from build123d import *

# Parameters (mm, degrees)
SKETCH1_R             = 6.477
BOSS_EXTRUDE1_DEPTH   = 5.08
BOSS_EXTRUDE1_2_DEPTH = 5.08
SKETCH2_R             = 6.35
BOSS_EXTRUDE2_DEPTH   = 12.7
SKETCH3_R             = 9.652
CUT_EXTRUDE1_DEPTH    = 3.81
SKETCH5_R             = 3.175


with BuildPart() as part:
    # Sketch1 → Boss-Extrude1 (new, symmetric)
    with BuildSketch(Plane(origin=(0, 0, 0), x_dir=(1, 0, 0), z_dir=(0, 1, 0))):
        with BuildLine():
            Line((-46.355, -19.05), (-46.355, -9.651164438))
            ThreePointArc((-46.355, -9.651164438), (-38.1, 12.7), (-29.845, -9.651164438))
            Line((-29.845, -9.651164438), (-29.845, -19.05))
            ThreePointArc((-29.845, -19.05), (-38.1, -27.305), (-46.355, -19.05))
        make_face()
        with Locations(Location((-38.1, 0, 0), (0, 0, 270))):
            Circle(SKETCH1_R, mode=Mode.SUBTRACT)
    extrude(amount=BOSS_EXTRUDE1_DEPTH, both=True)



with BuildPart() as body_2:
    # Sketch1 → Boss-Extrude1 2 (new, symmetric)
    with BuildSketch(Plane(origin=(0, 0, 0), x_dir=(1, 0, 0), z_dir=(0, 1, 0))):
        with BuildLine():
            Line((29.845, -19.05), (29.845, -9.651164438))
            ThreePointArc((29.845, -9.651164438), (38.1, 12.7), (46.355, -9.651164438))
            Line((46.355, -9.651164438), (46.355, -19.05))
            ThreePointArc((46.355, -19.05), (38.1, -27.305), (29.845, -19.05))
        make_face()
        with Locations(Location((38.1, 0, 0), (0, 0, 90))):
            Circle(SKETCH1_R, mode=Mode.SUBTRACT)
    extrude(amount=BOSS_EXTRUDE1_2_DEPTH, both=True)


with BuildPart() as part_1:
    add(part.part)

    add(body_2.part)  # Boss-Extrude2 merges body 2
    # Sketch2 → Boss-Extrude2 (add)
    with BuildSketch(Plane.XZ.offset(5.08)):
        with Locations(Location((-38.1, 19.05, 0), (0, 0, 270))):
            Circle(SKETCH2_R)
        with Locations(Location((38.1, 19.05, 0), (0, 0, 270))):
            Circle(SKETCH2_R)
    extrude(amount=BOSS_EXTRUDE2_DEPTH)

    # Sketch3 → Cut-Extrude1 (cut)
    with BuildSketch(Plane(origin=(0, 5.08, 0), x_dir=(1, 0, 0), z_dir=(0, 1, 0))):
        with Locations(Location((-38.1, 0, 0), (0, 0, 270))):
            Circle(SKETCH3_R)
        with Locations(Location((38.1, 0, 0), (0, 0, 270))):
            Circle(SKETCH3_R)
    extrude(amount=-CUT_EXTRUDE1_DEPTH, mode=Mode.SUBTRACT)

    # Sweep1: sweep along a path in Sketch6
    with BuildLine(Plane(origin=(0, 0, 0), x_dir=(1, 0, 0), z_dir=(0, 1, 0))) as sweep1_path:
        Line((38.1, 12.192), (38.1, 44.45))
        ThreePointArc((38.1, 44.45), (35.310192091, 51.185192091), (28.575, 53.975))
        Line((28.575, 53.975), (-28.575, 53.975))
        ThreePointArc((-28.575, 53.975), (-35.310192091, 51.185192091), (-38.1, 44.45))
        Line((-38.1, 44.45), (-38.1, 12.192))
    # Sketch5 → Sweep1 (sweep)
    with BuildSketch(Plane.XY.offset(-12.192)):
        with Locations((38.1, 0)):
            Circle(SKETCH5_R)
    sweep(path=sweep1_path.line)


solid = part_1.part
The listing builds one solid part. Answer for the finished solid, in the listing's coordinates (mm). A direction names the side the tool comes from. Give positions to 0.01 mm unless a question says otherwise; leave off trailing zeros. Write each loop counter-clockwise with the first axis right and the second up, starting at its lowest first coordinate (ties: lowest second). Pieces come first, ordered by that corner, then holes.
1) Section D-D (x = 6) is taken. Write down the section's boundary in (y, z) (3 decimals), and give its area (3 significant figures).
2) Find the intervals of material crossed by L1, parallel to X at y = 2.8, z = 0; L2, parallel to Z at x = -38.1, y = -3.25 (3 decimals); L3, parallel to X at y = -2, z = 0, in increasing order.
3) Section A-A (z = 17) is taken. Write down the section's boundary in (x, y) (3 decimals).
4) A tool of negligible diameter and unlimited length cuts with its end or side. For faces 1 (the face through (31.8, 1.27, -2.3)), 2 (the face through (-0.4, -0.1, -50.8)), 3 (the face through (31.9, -11.34, 20.43)), 4 (the face through (29.845, 0, 14)), from which of +Z, -Z, +X, -X, +Y, -Y can it reach the whole face along a straight path? Write none if from no direction.
5) Given P1, Ø3, axis at y = 0.5, z = 13, coming from the +X side (3 decimals); P2, Ø10.5, axis at y = 1.5, z = 13.5, coming from the +X side; P3, Ø10, axis at x = -26.5, y = -8.5, coming from the -Z side, each flat-ended and moving along its own axis, determine where each tip first touches the part or whether it passes through.
6) Section B-B (y = 0) is taken. Write down the section's boundary in (x, z) (3 decimals).
7) For a pull along X with two mould halves and no side action, classify faces 5 (the face through (-38, 5.08, 11)), 6 (the face through (-47.522, 3.202, -2.092)), 7 (the face through (46.355, 0, 14)), 8 (the face through (-46.355, 0, 14)) as pulls with the +X half, pulls with the -X half, needs draft (parallel to the pull), parting line crosses it, or undercut.
8) Section C-C (z = 0) is taken. Write down the section's boundary in (x, y), and give its area (3 significant figures).
Response:
1. outline: circle Ø6.35 at (0, -53.975)
1. area: 31.7 mm2
2. L1: x = -50.8 to -47.75, -28.45 to -25.4, 25.4 to 28.45, 47.75 to 50.8
2. L2: z = -12.7 to -6.477, 6.477 to 27.305
2. L3: x = -50.8 to -44.58, -31.62 to -25.4, 25.4 to 31.62, 44.58 to 50.8
3. outline: (-46.355, -5.08) - (-44.11, -5.08) - (-44.11, -17.78) - (-32.09, -17.78) - (-32.09, -5.08) - (-29.845, -5.08) - (-29.845, 5.08) - (-46.355, 5.08) - close; (29.845, -5.08) - (32.09, -5.08) - (32.09, -17.78) - (44.11, -17.78) - (44.11, -5.08) - (46.355, -5.08) - (46.355, 5.08) - (29.845, 5.08) - close
4. face 1: +Y
4. face 2: none
4. face 3: -Y
4. face 4: +Z, +Y, -Y
5. P1: stops at x = 46.355
5. P2: stops at x = 47.76
5. P3: stops at z = -9.9
6. outline: (-46.355, 9.651) arc R12.7 ccw to (-41.275, -12.297) - (-41.275, -44.45) arc R12.7 ccw to (-28.575, -57.15) - (28.575, -57.15) arc R12.7 ccw to (41.275, -44.45) - (41.275, -12.297) arc R12.7 ccw to (46.355, 9.651) - (46.355, 19.05) arc R8.255 ccw to (29.845, 19.05) - (29.845, 9.651) arc R12.7 ccw to (34.925, -12.297) - (34.925, -44.45) arc R6.35 cw to (28.575, -50.8) - (-28.575, -50.8) arc R6.35 cw to (-34.925, -44.45) - (-34.925, -12.297) arc R12.7 ccw to (-29.845, 9.651) - (-29.845, 19.05) arc R8.255 ccw to (-46.355, 19.05) - close; hole circle Ø12.954 at (-38.1, 0); hole circle Ø12.954 at (38.1, 0)
7. face 5: needs draft
7. face 6: undercut
7. face 7: pulls with the +X half
7. face 8: pulls with the -X half
8. outline: (-50.8, -5.08) - (-44.58, -5.08) - (-44.58, 1.27) - (-47.75, 1.27) - (-47.75, 5.08) - (-50.8, 5.08) - close; (-31.62, -5.08) - (-25.4, -5.08) - (-25.4, 5.08) - (-28.45, 5.08) - (-28.45, 1.27) - (-31.62, 1.27) - close; (25.4, -5.08) - (31.62, -5.08) - (31.62, 1.27) - (28.45, 1.27) - (28.45, 5.08) - (25.4, 5.08) - close; (44.58, -5.08) - (50.8, -5.08) - (50.8, 5.08) - (47.75, 5.08) - (47.75, 1.27) - (44.58, 1.27) - close
8. area: 205 mm2
